from build123d import *

# Parameters (mm, degrees)
BOSS_EXTRU_1_DEPTH           = 2.5
ESQUISSE2_W                  = 39.25
ESQUISSE2_H                  = 5
BOSS_EXTRU_2_DEPTH           = 8.6
ESQUISSE16_W                 = 1.8
ESQUISSE16_H                 = 2.5
D_GAGEMENT_M32_AT_2_COUNT    = 2
D_GAGEMENT_M32_AT_2_PITCH    = 42.597094971
D_GAGEMENT_M32_AT_3_COUNT    = 2
D_GAGEMENT_M32_AT_3_PITCH    = 76.2
D_GAGEMENT_M32_AT_4_COUNT    = 2
D_GAGEMENT_M32_AT_4_PITCH    = 85.194189943
ESQUISSE18_R                 = 2.7
ENL_V_MAT_EXTRU_2_DEPTH      = 3
ENL_V_MAT_EXTRU_3_DEPTH      = 1.5
ENL_V_MAT_EXTRU_4_DEPTH      = 159.680567493
ENL_V_MAT_EXTRU_4_DEPTH_BACK = 10
ESQUISSE21_R                 = 6
CHANFREIN2_SIZE              = 0.577350269
CHANFREIN2_SIZE_2            = 1
ESQUISSE22_W                 = 14
ESQUISSE22_H                 = 20
ENL_V_MAT_EXTRU_13_DEPTH     = 1.5


with BuildPart() as part:
    # Esquisse1 → Boss.-Extru.1 (new body)
    with BuildSketch(Plane.XY):
        Polygon((0, -85), (17, -102), (121.25, -102), (121.25, 5), (17, 5), (0, -12), align=None)
    extrude(amount=BOSS_EXTRU_1_DEPTH)

    # Esquisse2 → Boss.-Extru.2 (add)
    with BuildSketch(Plane.XY.offset(2.5)):
        Polygon((5, -82.928932188), (19.071067812, -97), (116.25, -97), (116.25, 0), (111.25, 0), (111.25, 5), (121.25, 5), (121.25, -102), (17, -102), (0, -85), (0, -12), (17, 5), (51, 5), (51, 0), (19.071067812, 0), (5, -14.071067812), align=None)
        with Locations((84.625, 2.5)):
            Rectangle(ESQUISSE2_W, ESQUISSE2_H)
    extrude(amount=BOSS_EXTRU_2_DEPTH)

    # Esquisse8 → Révolution3 (revolve)
    with BuildSketch(Plane(origin=(98.725, -41.37, 2.5), x_dir=(0, 0, -1), z_dir=(1, 0, 0)), mode=Mode.PRIVATE) as r_volution3_sk:
        Polygon((0, 1.75), (0, 7.75), (-2, 5.25), (-2, 1.75), align=None)
    revolve(r_volution3_sk.sketch.rotate(Axis((98.725, -41.37, 2.5), (0, 0, 1)), 90), axis=Axis((98.725, -41.37, 2.5), (0, 0, 1)))

    # Esquisse9 → Révolution4 (revolve)
    with BuildSketch(Plane(origin=(41.575, -79.47, 2.5), x_dir=(0, 0, -1), z_dir=(1, 0, 0)), mode=Mode.PRIVATE) as r_volution4_sk:
        Polygon((0, 1.75), (0, 7.75), (-2, 5.25), (-2, 1.75), align=None)
    revolve(r_volution4_sk.sketch.rotate(Axis((41.575, -79.47, 2.5), (0, 0, 1)), 90), axis=Axis((41.575, -79.47, 2.5), (0, 0, 1)))

    # Esquisse10 → Révolution5 (revolve)
    with BuildSketch(Plane(origin=(98.725, -79.47, 2.5), x_dir=(0, 0, -1), z_dir=(1, 0, 0)), mode=Mode.PRIVATE) as r_volution5_sk:
        Polygon((0, 1.75), (0, 7.75), (-2, 5.25), (-2, 1.75), align=None)
    revolve(r_volution5_sk.sketch.rotate(Axis((98.725, -79.47, 2.5), (0, 0, 1)), 90), axis=Axis((98.725, -79.47, 2.5), (0, 0, 1)))

    # Esquisse16 → Dégagement M32 (revolve, cut)
    with BuildSketch(Plane(origin=(22.525, -41.37, 2.5), x_dir=(0, -1, 0), z_dir=(1, 0, 0))):
        with Locations((0.9, 1.25)):
            Rectangle(ESQUISSE16_W, ESQUISSE16_H)
    d_gagement_m32 = revolve(axis=Axis((22.525, -41.37, 8.85), (0, 0, -1)), mode=Mode.SUBTRACT)

    # Dégagement M32 at 2: Dégagement M32 ×2
    with Locations(*[Vector(0.4472135954999577, -0.8944271909999161, 0) * (i * D_GAGEMENT_M32_AT_2_PITCH) for i in range(1, D_GAGEMENT_M32_AT_2_COUNT)]):
        add(d_gagement_m32, mode=Mode.SUBTRACT)

    # Dégagement M32 at 3: Dégagement M32 ×2
    with Locations(*[(i * D_GAGEMENT_M32_AT_3_PITCH, 0, 0) for i in range(1, D_GAGEMENT_M32_AT_3_COUNT)]):
        add(d_gagement_m32, mode=Mode.SUBTRACT)

    # Dégagement M32 at 4: Dégagement M32 ×2
    with Locations(*[Vector(0.8944271909999159, -0.44721359549995804, 0) * (i * D_GAGEMENT_M32_AT_4_PITCH) for i in range(1, D_GAGEMENT_M32_AT_4_COUNT)]):
        add(d_gagement_m32, mode=Mode.SUBTRACT)

    # Esquisse17 → Révolution6 (revolve)
    with BuildSketch(Plane(origin=(22.525, -41.37, 2.5), x_dir=(0, 0, -1), z_dir=(1, 0, 0)), mode=Mode.PRIVATE) as r_volution6_sk:
        Polygon((0, 1.75), (0, 7.75), (-2, 5.25), (-2, 1.75), align=None)
    revolve(r_volution6_sk.sketch.rotate(Axis((22.525, -41.37, 2.5), (0, 0, 1)), 90), axis=Axis((22.525, -41.37, 2.5), (0, 0, 1)))

    # Esquisse18 → Enlèv. mat.-Extru.2 (cut)
    with BuildSketch(Plane(origin=(0, 0, 0), x_dir=(-1, 0, 0), z_dir=(0, 0, -1))):
        with Locations((-22.525, -41.37)):
            Circle(ESQUISSE18_R)
        with Locations((-98.725, -41.37)):
            Circle(ESQUISSE18_R)
        with Locations((-41.575, -79.47)):
            Circle(ESQUISSE18_R)
        with Locations((-98.725, -79.47)):
            Circle(ESQUISSE18_R)
    extrude(amount=-ENL_V_MAT_EXTRU_2_DEPTH, mode=Mode.SUBTRACT)

    # Esquisse20 → Enlèv. mat.-Extru.3 (cut)
    with BuildSketch(Plane.XY.offset(11.1)):
        Polygon((119.75, 2.5), (18.035533906, 2.5), (1.5, -14.035533906), (1.5, -84.095836944), (17.904163056, -100.5), (119.75, -100.5), align=None)
    extrude(amount=-ENL_V_MAT_EXTRU_3_DEPTH, mode=Mode.SUBTRACT)

    # Esquisse21 → Enlèv. mat.-Extru.4 (cut, two sides: drawn at the far end of the back side and taken through both)
    with BuildSketch(Plane.XY.offset(2.5).offset(-ENL_V_MAT_EXTRU_4_DEPTH_BACK)):
        with Locations(Location((98.725, -27.87, 0), (0, 0, 180))):
            Circle(ESQUISSE21_R)
        with Locations(Location((41.525, -27.37, 0), (0, 0, 180))):
            Circle(ESQUISSE21_R)
        with Locations(Location((79.725, -83.97, 0), (0, 0, 180))):
            Circle(ESQUISSE21_R)
    extrude(amount=ENL_V_MAT_EXTRU_4_DEPTH + ENL_V_MAT_EXTRU_4_DEPTH_BACK, mode=Mode.SUBTRACT)

    # Chanfrein2
    # the kernel refuses this chamfer: 1, 0.577350269 mm, written as the material it adds along each edge
    with BuildSketch(Plane(origin=(98.725, -79.47, 3), x_dir=(-1, 0, 0), z_dir=(0, -1, 0))) as chanfrein2_piece_1_section:
        Polygon((2.7, CHANFREIN2_SIZE), (2.7 - CHANFREIN2_SIZE_2, 0), (2.7, 0), align=None)
    chanfrein2_piece_1 = revolve(axis=Axis((98.725, -79.47, 3), (0, 0, -1)), mode=Mode.PRIVATE)
    chanfrein2_piece_1 = chanfrein2_piece_1 - Plane(origin=(98.725, -79.47, 2.701530762), x_dir=(-1, 0, 0), z_dir=(0, 0, -1)) * Cylinder(1.75, 11, mode=Mode.PRIVATE)
    add(chanfrein2_piece_1)
    with BuildSketch(Plane(origin=(41.575, -79.47, 3), x_dir=(-1, 0, 0), z_dir=(0, -1, 0))) as chanfrein2_piece_2_section:
        Polygon((2.7, CHANFREIN2_SIZE), (2.7 - CHANFREIN2_SIZE_2, 0), (2.7, 0), align=None)
    chanfrein2_piece_2 = revolve(axis=Axis((41.575, -79.47, 3), (0, 0, -1)), mode=Mode.PRIVATE)
    chanfrein2_piece_2 = chanfrein2_piece_2 - Plane(origin=(41.575, -79.47, 2.701530762), x_dir=(-1, 0, 0), z_dir=(0, 0, -1)) * Cylinder(1.75, 11, mode=Mode.PRIVATE)
    add(chanfrein2_piece_2)
    with BuildSketch(Plane(origin=(22.525, -41.37, 3), x_dir=(-1, 0, 0), z_dir=(0, -1, 0))) as chanfrein2_piece_3_section:
        Polygon((2.7, CHANFREIN2_SIZE), (2.7 - CHANFREIN2_SIZE_2, 0), (2.7, 0), align=None)
    chanfrein2_piece_3 = revolve(axis=Axis((22.525, -41.37, 3), (0, 0, -1)), mode=Mode.PRIVATE)
    chanfrein2_piece_3 = chanfrein2_piece_3 - Plane(origin=(22.525, -41.37, 2.701530762), x_dir=(-1, 0, 0), z_dir=(0, 0, -1)) * Cylinder(1.75, 11, mode=Mode.PRIVATE)
    add(chanfrein2_piece_3)
    with BuildSketch(Plane(origin=(98.725, -41.37, 3), x_dir=(-1, 0, 0), z_dir=(0, -1, 0))) as chanfrein2_piece_4_section:
        Polygon((2.7, CHANFREIN2_SIZE), (2.7 - CHANFREIN2_SIZE_2, 0), (2.7, 0), align=None)
    chanfrein2_piece_4 = revolve(axis=Axis((98.725, -41.37, 3), (0, 0, -1)), mode=Mode.PRIVATE)
    chanfrein2_piece_4 = chanfrein2_piece_4 - Plane(origin=(98.725, -41.37, 2.701530762), x_dir=(-1, 0, 0), z_dir=(0, 0, -1)) * Cylinder(1.75, 11, mode=Mode.PRIVATE)
    add(chanfrein2_piece_4)

    # Esquisse22 → Enlèv. mat.-Extru.13 (cut)
    with BuildSketch(Plane.XY.offset(2.5)):
        with Locations((34.525, -11.27)):
            Rectangle(ESQUISSE22_W, ESQUISSE22_H)
    extrude(amount=-ENL_V_MAT_EXTRU_13_DEPTH, mode=Mode.SUBTRACT)


solid = part.part
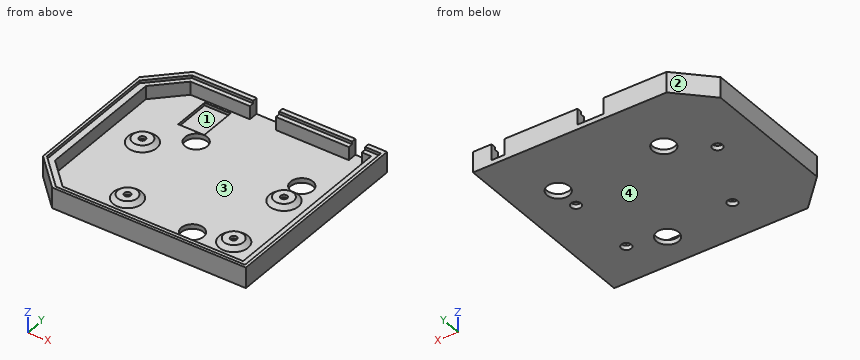
Could you check a few things on this model? Use its own coordinates, in mm. Face numbers are marked on the shaded views. Coordinates: 2 decimals unless noted, no trailing zeros. Loops run counter-clockwise (first coordinate to the right, second up) from the corner with the lowest first, then second, coordinate; pieces in that order, holes last.
1. We'd pull the mould along X, two halves only. Please class the marked faces 1, 2, 3 and 4: released by +X, released by -X, zero draft, split by the parting line, or undercut.
2. For P1, Ø4.5, axis at x = 41.575, y = -79.47, coming from the +Z side; P2, Ø4, axis at x = 98.5, y = -88.5, coming from the -Z side; P3, Ø2, axis at x = 22.525, y = -41.37, coming from the -Z side; P4, Ø4.5, axis at x = 98.725, y = -41.37, coming from the -Z side, each with a flat end and sliding along its axis, tell me the tip position at first contact or that it passes through.
3. Imagine slicing it at D-D (y = -41.37). Give the number of separate pieces and of enclosed holes in the cut face, and give its area (3 significant figures).
4. Imagine slicing it at A-A (z = 6.25). Please give me the cut outline in (x, y), and give its area (3 significant figures).
5. Imagine slicing it at B-B (y = -69.5). Please give me the cut outline in (x, z), and give its area (3 significant figures).
6. I need wall thicknesses on L1, parallel to X at y = -27.87, z = 0.8 (3 decimals); L2, parallel to X at y = -31.5, z = 5; L3, parallel to Y at x = 83, z = 7.75. Which ranges of each line are inside material? Lowest first, please.
7. Imagine slicing it at C-C (x = 67). Please give me the cut outline in (y, z), and give its area (4 significant figures).
Computed values:
1. face 1: undercut
1. face 2: released by -X
1. face 3: undercut
1. face 4: zero draft
2. P1: stops at z = 4.5
2. P2: stops at z = 0
2. P3: passes through
2. P4: stops at z = 2.68
3. separate pieces: 3
3. enclosed holes: 0
3. area: 389 mm2
4. outline: (0, -85) - (17, -102) - (121.25, -102) - (121.25, 5) - (111.25, 5) - (111.25, 0) - (116.25, 0) - (116.25, -97) - (19.07, -97) - (5, -82.93) - (5, -14.07) - (19.07, 0) - (51, 0) - (51, 5) - (17, 5) - (0, -12) - close; (65, 0) - (104.25, 0) - (104.25, 5) - (65, 5) - close
4. area: 1,990 mm2
5. outline: (0, 0) - (121.25, 0) - (121.25, 11.1) - (119.75, 11.1) - (119.75, 9.6) - (116.25, 9.6) - (116.25, 2.5) - (5, 2.5) - (5, 9.6) - (1.5, 9.6) - (1.5, 11.1) - (0, 11.1) - close
5. area: 379 mm2
6. L1: x = 0 to 35.546, 47.504 to 92.725, 104.725 to 121.25
6. L2: x = 0 to 5, 116.25 to 121.25
6. L3: y = -102 to -97, 0 to 5
7. outline: (-102, 0) - (5, 0) - (5, 11.1) - (2.5, 11.1) - (2.5, 9.6) - (0, 9.6) - (0, 2.5) - (-97, 2.5) - (-97, 9.6) - (-100.5, 9.6) - (-100.5, 11.1) - (-102, 11.1) - close
7. area: 344.5 mm2
